Verification items for the finished model (mm, model axes). A direction names the side the tool comes from. Round coordinates to 2 decimals unless told otherwise and drop trailing zeros. Order: outer loops, then holes, each group sorted by start corner. A loop starts at its lowest first (then second) coordinate and runs counter-clockwise, first axis right, second up. Notation, with made-up numbers: (71, 28) -> (112, 28) arc R19 cw to (112, 55) -> close; hole circle Ø8 at (33, 48). An arc over 180 degrees is marked (long way). Put each result on its own line as item: value.
```python
from build123d import *

# Parameters (mm, degrees)
SKETCH059_W          = 20
SKETCH059_H          = 20
PAD020_DEPTH         = 3
SKETCH060_W          = 9
SKETCH060_H          = 6.2
POCKET042_DEPTH      = 3.001
CHAMFER019_SIZE      = 2
PAD021_DEPTH         = 3
SKETCH062_R          = 2
PAD022_DEPTH         = 3
CHAMFER020_SIZE      = 0.4
SKETCH063_W          = 5.5
SKETCH063_H          = 20
PAD023_DEPTH         = 12
FILLET012_R          = 6
FILLET013_R          = 2
SKETCH064_R          = 1.6
POCKET043_DEPTH      = 10.001
POCKET043_DEPTH_BACK = 10.001
CHAMFER021_SIZE      = 2
POCKET044_DEPTH      = 3
CHAMFER022_SIZE      = 0.5


with BuildPart() as part:
    # Sketch059 → Pad020 (new body)
    with BuildSketch(Plane.YZ):
        Rectangle(SKETCH059_W, SKETCH059_H)
    extrude(amount=-PAD020_DEPTH)

    # Sketch060 (on Face5 of Pad020) → Pocket042 (cut, through all)
    with BuildSketch(Plane.YZ):
        with Locations((0, -6.9)):
            Rectangle(SKETCH060_W, SKETCH060_H)
        with Locations((0, 6.9)):
            Rectangle(SKETCH060_W, SKETCH060_H)
    extrude(amount=-POCKET042_DEPTH, mode=Mode.SUBTRACT)

    # Chamfer019
    chamfer019_edges = [part.edges().sort_by_distance(p)[0] for p in [
        (-1.5, 4.5, -3.8),
        (-1.5, -4.5, -3.8),
        (-1.5, -4.5, 3.8),
        (-1.5, 4.5, 3.8),
    ]]
    chamfer(chamfer019_edges, length=CHAMFER019_SIZE)

    # Sketch061 (on Face1 of Chamfer019) → Pad021 (join)
    with BuildSketch(Plane.YZ):
        Polygon((-10, 3), (-4.35, 3), (-4.1, 2.75), (-4.1, -2.75), (-4.35, -3), (-10, -3), align=None)
    pad021 = extrude(amount=PAD021_DEPTH)

    # Mirrored001: Pad021 across Sketch061 V_Axis
    add(pad021.mirror(Plane(origin=(0, 0, 0), x_dir=(1, 0, 0), z_dir=(0, 1, 0))))

    # Sketch062 (on Face1 of Mirrored001) → Pad022 (join)
    with BuildSketch(Plane.YZ):
        Circle(SKETCH062_R)
    extrude(amount=PAD022_DEPTH)

    # Chamfer020
    chamfer020_edges = [part.edges().sort_by_distance(p)[0] for p in [
        (3, -2, 0),
        (3, -7.175, 3),
        (3, -4.225, 2.875),
        (3, -4.1, 0),
        (3, -4.225, -2.875),
        (3, -7.175, -3),
        (3, -10, 0),
        (3, 7.175, 3),
        (3, 4.225, 2.875),
        (3, 4.1, 0),
        (3, 4.225, -2.875),
        (3, 7.175, -3),
        (3, 10, 0),
    ]]
    chamfer(chamfer020_edges, length=CHAMFER020_SIZE)

    # Sketch063 (on Face7 of Chamfer020) → Pad023 (join)
    with BuildSketch(Plane(origin=(-3, 0, 0), x_dir=(0, -1, 0), z_dir=(-1, 0, 0))):
        with Locations((-7.25, 0)):
            Rectangle(SKETCH063_W, SKETCH063_H)
        with Locations((7.25, 0)):
            Rectangle(SKETCH063_W, SKETCH063_H)
    extrude(amount=PAD023_DEPTH)

    # Fillet012
    fillet012_edges = [part.edges().sort_by_distance(p)[0] for p in [
        (-15, 7.25, -10),
        (-15, -7.25, -10),
        (-15, -7.25, 10),
        (-15, 7.25, 10),
    ]]
    fillet(fillet012_edges, radius=FILLET012_R)

    # Fillet013
    fillet013_edges = [part.edges().sort_by_distance(p)[0] for p in [
        (-3, 0, 3.8),
        (-3, 0, -3.8),
        (-3, 3.5, 4.8),
        (-3, -3.5, 4.8),
        (-3, -3.5, -4.8),
        (-3, 3.5, -4.8),
    ]]
    fillet(fillet013_edges, radius=FILLET013_R)

    # Sketch064 → Pocket043 (cut, two sides)
    with BuildSketch(Plane.XZ) as pocket043_sk:
        with Locations((-9, 0)):
            Circle(SKETCH064_R)
    extrude(amount=-POCKET043_DEPTH, mode=Mode.SUBTRACT)
    extrude(pocket043_sk.sketch, amount=POCKET043_DEPTH_BACK, mode=Mode.SUBTRACT)

    # Chamfer021
    chamfer021_edges = [part.edges().sort_by_distance(p)[0] for p in [
        (-10.6, 10, 0),
    ]]
    chamfer(chamfer021_edges, length=CHAMFER021_SIZE)

    # Sketch065 (on Face26 of Chamfer021) → Pocket044 (cut)
    with BuildSketch(Plane.XZ.offset(10)):
        Polygon((-5.778385, 0), (-7.389193, 2.79), (-10.610807, 2.79), (-12.221615, 0), (-10.610807, -2.79), (-7.389193, -2.79), align=None)
    extrude(amount=-POCKET044_DEPTH, mode=Mode.SUBTRACT)

    # Chamfer022
    chamfer022_edges = [part.edges().sort_by_distance(p)[0] for p in [
        (-4.5, -10, 10),
        (-4.5, 10, 10),
        (-4.5, -4.5, 10),
        (-4.5, 4.5, 10),
        (-10.6, 4.5, 0),
        (-10.6, -4.5, 0),
        (-10.6, -7, 0),
    ]]
    chamfer(chamfer022_edges, length=CHAMFER022_SIZE)


with BuildPart() as part_1:
    # Body012 placement: moved
    add(part.part.moved(Location((-154, 26.5, 285))))


solid = part_1.part
```
Item 1: Sectioned sample at A-A, the plane x = -158.25. Record the boundary of the cut face in (y, z).
Geometry check:
outline: (16.5, 275.5) -> (17, 275) -> (21.5, 275) -> (22, 275.5) -> (22, 294.5) -> (21.5, 295) -> (17, 295) -> (16.5, 294.5) -> close; (31, 275.5) -> (31.5, 275) -> (36, 275) -> (36.5, 275.5) -> (36.5, 294.5) -> (36, 295) -> (31.5, 295) -> (31, 294.5) -> close
Item 2: Sectioned sample at C-C, the plane x = -153. Record the boundary of the cut face in (y, z), then the cut area to 3 significant figures.
Geometry check:
outline: (16.5, 282) -> (22.15, 282) -> (22.4, 282.25) -> (22.4, 287.75) -> (22.15, 288) -> (16.5, 288) -> close; circle Ø4 at (26.5, 285); (30.6, 282.25) -> (30.85, 282) -> (36.5, 282) -> (36.5, 288) -> (30.85, 288) -> (30.6, 287.75) -> close
area: 83.2 mm2
Item 3: Release check for a two-part mould opening along Z. For faces 1 (the face through (-153, 19, 282)), 2 (the face through (-167.033, 31.142, 292.946)), 3 (the face through (-165.427, 17.979, 283.625)) record: pulls with the +Z half, pulls with the -Z half, needs draft (parallel to the pull), parting line crosses it, or undercut.
Geometry check:
face 1: pulls with the -Z half
face 2: pulls with the +Z half
face 3: undercut
Item 4: Depth check by flat-ended pin: pin 1 Ø1.3 at (x, y) = (-153, 32.5) entering from -Z; pin 2 Ø2 at (x, y) = (-156, 26) entering from -Z; pin 3 Ø3 at (y, z) = (25, 283.5) entering from -X. Enter the tip coordinate at first touch or a pass-through.
Geometry check:
pin 1: z = 282
pin 2: z = 281.2
pin 3: x = -157
Item 5: Material ranges on line 1 along Z through (x, y) = (-163, 33.2); line 2 along X through (y, z) = (32.55, 285); line 3 along Y through (x, z) = (-162.25, 279.75), recorded low to high.
Geometry check:
line 1: 275 to 283.4, 286.6 to 295
line 2: -169 to -164.6, -161.4 to -151
line 3: 16.5 to 22, 31 to 36.5
Item 6: Sectioned sample at B-B, the plane y = 33.5. Record the boundary of the cut face in (x, z), then the cut area to 3 significant figures.
Geometry check:
outline: (-169, 281) arc R6 ccw to (-163, 275) -> (-154, 275) -> (-154, 282) -> (-151.4, 282) -> (-151, 282.4) -> (-151, 287.6) -> (-151.4, 288) -> (-154, 288) -> (-154, 295) -> (-163, 295) arc R6 ccw to (-169, 289) -> close; hole circle Ø3.2 at (-163, 285)
area: 294 mm2
Item 7: Tool access check on faces 4 (the face through (-156.399, 30.092, 280.914)), 5 (the face through (-161.6, 19.5, 283.2)), 6 (the face through (-154.5, 26.5, 281.2)). Record the directions out of +Z, -Z, +X, -X, +Y, -Y that give a thin tool (end or side, any length) a straight path to the whole face; none if there is none.
Geometry check:
face 4: -Z, -X
face 5: -Y
face 6: -Z, +X, -X
Item 8: Sectioned sample at D-D, the plane y = 26.5. Record the boundary of the cut face in (x, z), then the cut area to 3 significant figures.
Geometry check:
outline: (-157, 283.2) arc R2 ccw to (-155, 281.2) -> (-154, 281.2) -> (-154, 283) -> (-151.4, 283) -> (-151, 283.4) -> (-151, 286.6) -> (-151.4, 287) -> (-154, 287) -> (-154, 288.8) -> (-155, 288.8) arc R2 ccw to (-157, 286.8) -> close
area: 32.9 mm2
